Verification items for the finished model (mm, model axes). A direction names the side the tool comes from. Give positions to 0.01 mm unless a question says otherwise; leave off trailing zeros. Order: outer loops, then holes, each group sorted by start corner. A loop starts at its lowest first (then second) coordinate and runs counter-clockwise, first axis right, second up. Notation, with made-up numbers: (7.5, 18.25) - (51.5, 18.25) arc R24 ccw to (51.5, 43.25) - close; hole circle Ø5 at (-0.5, 86.25). An arc over 180 degrees is marked (long way). Answer as a JSON object with one key per item and string values.
```python
from build123d import *

# Parameters (mm, degrees)
BOSS_EXTRUDE1_DEPTH = 101.6
SKETCH2_R           = 2.4892
CUT_EXTRUDE1_DEPTH  = 51.8


with BuildPart() as part:
    # Sketch1 → Boss-Extrude1 (new body)
    with BuildSketch(Plane(origin=(0, 0, 0), x_dir=(1, 0, 0), z_dir=(0, 1, 0))):
        Polygon((0, 0), (25.4, 0), (25.4, 3.175), (3.175, 3.175), (3.175, 47.625), (25.4, 47.625), (25.4, 50.8), (0, 50.8), align=None)
    extrude(amount=BOSS_EXTRUDE1_DEPTH)

    # Sketch2 → Cut-Extrude1 (cut, through all)
    with BuildSketch(Plane(origin=(0, 0, -50.8), x_dir=(-1, 0, 0), z_dir=(0, 0, -1))):
        with Locations((-12.7, 12.7)):
            Circle(SKETCH2_R)
        with Locations((-12.7, 95.25)):
            Circle(SKETCH2_R)
        with Locations((-12.7, 82.55)):
            Circle(SKETCH2_R)
    extrude(amount=-CUT_EXTRUDE1_DEPTH, mode=Mode.SUBTRACT)


solid = part.part
```
(1) Access from +Z, -Z, +X, -X, +Y, -Y to the whole of each face (thin tool, end or side, straight path). Record for faces 4 (the flat face through (14, 50, -3.175)), 5 (the flat face through (2, 101.6, -26)).
Computed values:
{"face 4": "+X, +Y, -Y", "face 5": "+Z, -Z, +X, -X, +Y"}
(2) Section check D-D (y = 65.5). Record the cut outline in (x, z) (3 decimals), then the cut area to 3 significant figures.
Computed values:
{"outline": "(0, -50.8) - (25.4, -50.8) - (25.4, -47.625) - (3.175, -47.625) - (3.175, -3.175) - (25.4, -3.175) - (25.4, 0) - (0, 0) - close", "area": "302 mm²"}
(3) Section check B-B (x = 12.7). Count the separate pieces of the cut face and the enclosed holes in it, then the cut area to 3 significant figures.
Computed values:
{"separate pieces": "8", "enclosed holes": "0", "area": "550 mm²"}
(4) Release check for a two-part mould opening along Z. For faces 1 (the flat face through (14, 50, -47.625)), 2 (the flat face through (13, 50, 0)), 3 (the flat face through (13, 50, -50.8)) record: pulls with the +Z half, pulls with the -Z half, needs draft (parallel to the pull), parting line crosses it, or undercut.
Computed values:
{"face 1": "undercut", "face 2": "pulls with the +Z half", "face 3": "pulls with the -Z half"}
(5) Gauge pin test, flat ends, axial feed: pin 1 Ø22 at (y, z) = (37.5, -18.5) entering from +X (3 decimals); pin 2 Ø12 at (x, z) = (9.5, -32.5) entering from -Y. Record the tip position at first contact, or that the pin passes through.
Computed values:
{"pin 1": "stops at x = 3.175", "pin 2": "passes through"}
(6) Material ranges on line 1 along Y through (x, z) = (12.7, -48.9); line 2 along Z through (x, y) = (16, 22) (3 decimals); line 3 along X through (y, z) = (33, -27) (3 decimals), recorded low to high. Write a range as [from, to].
Computed values:
{"line 1": "y = [0, 10.21], [15.19, 80.06], [85.04, 92.76], [97.74, 101.6]", "line 2": "z = [-50.8, -47.625], [-3.175, 0]", "line 3": "x = [0, 3.175]"}
(7) Section check C-C (x = 19.25). Record the cut outline in (y, z) (3 decimals), then the cut area to 3 significant figures.
Computed values:
{"outline": "(0, -50.8) - (101.6, -50.8) - (101.6, -47.625) - (0, -47.625) - close; (0, -3.175) - (101.6, -3.175) - (101.6, 0) - (0, 0) - close", "area": "645 mm²"}
(8) Section check A-A (y = 12.7). Record the cut outline in (x, z) (3 decimals).
Computed values:
{"outline": "(0, -50.8) - (10.211, -50.8) - (10.211, -47.625) - (3.175, -47.625) - (3.175, -3.175) - (10.211, -3.175) - (10.211, 0) - (0, 0) - close; (15.189, -50.8) - (25.4, -50.8) - (25.4, -47.625) - (15.189, -47.625) - close; (15.189, -3.175) - (25.4, -3.175) - (25.4, 0) - (15.189, 0) - close"}
